from build123d import *

# Parameters (mm, degrees)
SKETCH1_W           = 218
SKETCH1_H           = 143
BOSS_EXTRUDE1_DEPTH = 101
FILLET1_R           = 6
SHELL1_START        = -103
SHELL1_OUTLINE_W    = 95
SHELL1_OUTLINE_H    = 131
SHELL1_DEPTH        = 206
SKETCH2_R           = 5
SKETCH2_R_2         = 2.925
CUT_EXTRUDE1_DEPTH  = 165.906791855


# Read off the part's stored shape, not the designer's step: Shell1
with BuildPart() as part:
    # Sketch1 → Boss-Extrude1 (new body)
    with BuildSketch(Plane(origin=(0, 0, 0), x_dir=(1, 0, 0), z_dir=(0, 1, 0))):
        Rectangle(SKETCH1_W, SKETCH1_H)
    extrude(amount=BOSS_EXTRUDE1_DEPTH)

    # Fillet1
    fillet1_edges = [part.edges().sort_by_distance(p)[0] for p in [
        (-109, 101, 0),
        (0, 101, 71.5),
        (109, 101, 0),
        (109, 50.5, 71.5),
        (-109, 50.5, 71.5),
        (-109, 50.5, -71.5),
        (109, 50.5, -71.5),
        (0, 101, -71.5),
    ]]
    fillet(fillet1_edges, radius=FILLET1_R)

    # Shell1 outline → Shell1 (cut)
    with BuildSketch(Plane.YZ.offset(SHELL1_START)):
        with Locations((47.5, 0)):
            Rectangle(SHELL1_OUTLINE_W, SHELL1_OUTLINE_H)
    extrude(amount=SHELL1_DEPTH, mode=Mode.SUBTRACT)

    # Sketch2 → Cut-Extrude1 (cut, through all)
    with BuildSketch(Plane(origin=(0, 101, 0), x_dir=(1, 0, 0), z_dir=(0, 1, 0))):
        with Locations(Location((-52.4, 0, 0), (0, 0, 270))):
            Circle(SKETCH2_R)
        with Locations(Location((-52.4, 35.525, 0), (0, 0, 270))):
            Circle(SKETCH2_R_2)
        with Locations(Location((-87.925, 0, 0), (0, 0, 270))):
            Circle(SKETCH2_R_2)
        with Locations(Location((-52.4, -35.525, 0), (0, 0, 270))):
            Circle(SKETCH2_R_2)
        with Locations(Location((-16.875, 0, 0), (0, 0, 270))):
            Circle(SKETCH2_R_2)
    extrude(amount=-CUT_EXTRUDE1_DEPTH, mode=Mode.SUBTRACT)


solid = part.part
Geometry: final body of the model. Coordinates: model frame, mm. A direction names the side the tool comes from. Give positions to 0.01 mm unless a question says otherwise; leave off trailing zeros. Loops run counter-clockwise (first coordinate to the right, second up) from the corner with the lowest first, then second, coordinate; pieces in that order, holes last. Notation, with made-up numbers: M 41.5,1.25 L 52.5,1.25 A24 ccw 52.5,18.25 Z; hole C 61.5,-10 d8. An arc over 180 degrees is marked long. Put each result on its own line as item: value. Start each with the question number.
1) Cut plane C-C (y = 44.5). Output: boundary loops of the cut face in (x, z).
2) Cut plane B-B (x = -52.4). Output: boundary loops of the cut face in (y, z).
3) Cut plane A-A (z = 0). Output: boundary loops of the cut face in (x, y).
4) Contact query for flat-ended pins moving along their axis: pin 1 (8 mm diameter, centred on x = -52.4, z = 0, fed in from -Y); pin 2 (6.5 mm diameter, centred on x = -52.4, z = 35.525, fed in from -Y). Output: stop coordinate, or through.
5) Cut plane D-D (z = 54.5). Output: boundary loops of the cut face in (x, y), then the cut area to 3 significant figures.
6) Pull-direction query (Z, two-part tool) for faces 3 (the cylindrical face through (1.442, 99.196, -69.789)), 4 (the flat face through (-1, 47, 65.5)), 5 (the flat face through (-109, 47, 1)); classes: pulls with the +Z half, pulls with the -Z half, needs draft (parallel to the pull), parting line crosses it, or undercut.
7) Access query for faces 1 (the cylindrical face through (-107.289, 48.165, -69.696)), 2 (the flat face through (-1, 47, -65.5)). Directions: +Z, -Z, +X, -X, +Y, -Y. A direction counts if a zero-diameter tool reaches every point of the face in a straight line with its end or side. Return the directions, or none.
8) Ray query, line 1 along Z through (x, y) = (0, 26); line 2 along X through (y, z) = (56.5, 54.5); line 3 along Z through (x, y) = (-52, 97). Return the intervals inside material, ascending.
Verdict:
1. outline: M -109,-65.5 A6 ccw -103,-71.5 L 103,-71.5 A6 ccw 109,-65.5 L 109,65.5 A6 ccw 103,71.5 L -103,71.5 A6 ccw -109,65.5 Z; hole M -103,-65.5 L 103,-65.5 L 103,65.5 L -103,65.5 Z
2. outline: M 0,-71.5 L 95,-71.5 A6 ccw 101,-65.5 L 101,-38.45 L 95,-38.45 L 95,-65.5 L 0,-65.5 Z; M 0,65.5 L 95,65.5 L 95,38.45 L 101,38.45 L 101,65.5 A6 ccw 95,71.5 L 0,71.5 Z; M 95,-32.6 L 101,-32.6 L 101,-5 L 95,-5 Z; M 95,5 L 101,5 L 101,32.6 L 95,32.6 Z
3. outline: M -109,0 L -103,0 L -103,95 L -90.85,95 L -90.85,101 L -103,101 A6 ccw -109,95 Z; M -85,95 L -57.4,95 L -57.4,101 L -85,101 Z; M -47.4,95 L -19.8,95 L -19.8,101 L -47.4,101 Z; M -13.95,95 L 103,95 L 103,0 L 109,0 L 109,95 A6 ccw 103,101 L -13.95,101 Z
4. pin 1: through
4. pin 2: y = 95
5. outline: M -109,0 L -103,0 L -103,95 L 103,95 L 103,0 L 109,0 L 109,95 A6 ccw 103,101 L -103,101 A6 ccw -109,95 Z
5. area: 2,430 mm2
6. face 3: pulls with the -Z half
6. face 4: undercut
6. face 5: needs draft
7. face 1: -Z, -X, +Y, -Y
7. face 2: -Y
8. line 1: -71.5 to -65.5, 65.5 to 71.5
8. line 2: -109 to -103, 103 to 109
8. line 3: -71.16 to -38.42, -32.63 to -4.98, 4.98 to 32.63, 38.42 to 71.16
